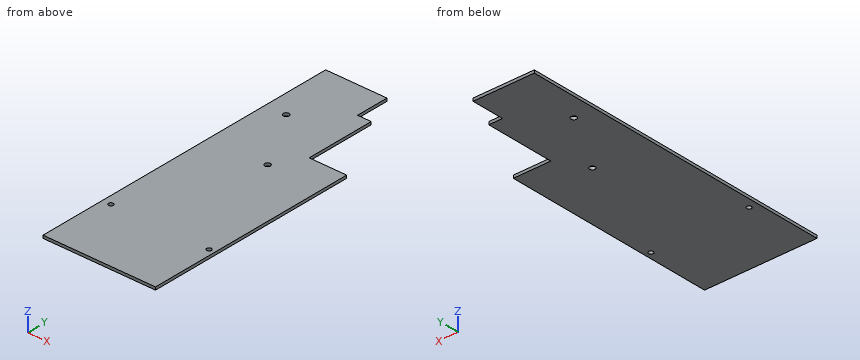
from build123d import *

# Parameters (mm, degrees)
RESSALTO_EXTRUS_O1_DEPTH                   = 1.5
CORTE_EXTRUS_O2_REACH                      = 167.453
ESBO_O5_R                                  = 1.5
BROCA_DE_ROSQUEAR_PARA_TARRAXA_DE_M3X0_5_D = 2.5
CORTE_EXTRUS_O3_REACH                      = 167.453
ESBO_O15_R                                 = 1.5
CORTE_EXTRUS_O4_REACH                      = 167.453
ESBO_O16_W                                 = 7.289764361
ESBO_O16_H                                 = 17.697498775


with BuildPart() as part:
    # Esboço2 → Ressalto-extrusão1 (new body)
    with BuildSketch(Plane(origin=(0, 0, 25.401562241), x_dir=(-1, 0, 0), z_dir=(0, 0, -1))):
        Polygon((40, 9.462441068), (0, 9.462441068), (0, -45.537558932), (-20, -45.537558932), (-20, -160.537558932), (40, -160.537558932), align=None)
    extrude(amount=RESSALTO_EXTRUS_O1_DEPTH)

    # Esboço5 → Corte-extrusão2 (cut, up to next)
    with BuildSketch(Plane(origin=(0, 0, 23.901562241), x_dir=(-1, 0, 0), z_dir=(0, 0, -1)), mode=Mode.PRIVATE) as corte_extrus_o2_sk1:
        with Locations((28.9, -26.787558932)):
            Circle(ESBO_O5_R)
    corte_extrus_o2_tool1 = extrude(corte_extrus_o2_sk1.sketch, amount=-CORTE_EXTRUS_O2_REACH, mode=Mode.PRIVATE) & part.part
    add(corte_extrus_o2_tool1.solids().sort_by_distance((-28.9, -26.787559, 23.901562))[0], mode=Mode.SUBTRACT)

    # Broca de rosquear para tarraxa de M3x0.52 (through all)
    with Locations(Plane(origin=(0, 0, 23.901562241), x_dir=(-1, 0, 0), z_dir=(0, 0, -1))):
        with Locations((-16.849169709, -124.734682683), (35.5, -124.808922584)):
            Hole(BROCA_DE_ROSQUEAR_PARA_TARRAXA_DE_M3X0_5_D / 2)

    # Esboço15 → Corte-extrusão3 (cut, up to next)
    with BuildSketch(Plane(origin=(0, 0, 23.901562241), x_dir=(-1, 0, 0), z_dir=(0, 0, -1)), mode=Mode.PRIVATE) as corte_extrus_o3_sk1:
        with Locations((8.9, -60.537558932)):
            Circle(ESBO_O15_R)
    corte_extrus_o3_tool1 = extrude(corte_extrus_o3_sk1.sketch, amount=-CORTE_EXTRUS_O3_REACH, mode=Mode.PRIVATE) & part.part
    add(corte_extrus_o3_tool1.solids().sort_by_distance((-8.9, -60.537559, 23.901562))[0], mode=Mode.SUBTRACT)

    # Esboço16 → Corte-extrusão4 (cut, up to next)
    with BuildSketch(Plane(origin=(0, 0, 23.901562241), x_dir=(-1, 0, 0), z_dir=(0, 0, -1)), mode=Mode.PRIVATE) as corte_extrus_o4_sk1:
        with Locations((3.644882181, 0.61369168)):
            Rectangle(ESBO_O16_W, ESBO_O16_H)
    corte_extrus_o4_tool1 = extrude(corte_extrus_o4_sk1.sketch, amount=-CORTE_EXTRUS_O4_REACH, mode=Mode.PRIVATE) & part.part
    add(corte_extrus_o4_tool1.solids().sort_by_distance((-3.644882, 0.613692, 23.901562))[0], mode=Mode.SUBTRACT)


solid = part.part
Work out the finished part from the listing and answer in its coordinate system (mm). Round coordinates to 2 decimals unless told otherwise and drop trailing zeros. Write each loop counter-clockwise with the first axis right and the second up, starting at its lowest first coordinate (ties: lowest second). Pieces come first, ordered by that corner, then holes. Notation, with made-up numbers: (-39, -34.5) -> (-10, -34.5) arc R13 cw to (-10, -27.5) -> close; hole circle Ø8 at (-34.75, 3). An arc over 180 degrees is marked (long way). Answer as CSV lines item,"result". Start each with the question number.
(1) The part is cut by section C-C, the plane y = -18.5. Give the vertices of the cut face in (x, z), then the cut area to 3 significant figures.
(2) Each of these flat-tipped pins is pushed along its axis until it touches: pin 1 (0.8 mm diameter, centred on x = 7, z = 24.5, fed in from +Y); pin 2 (2 mm diameter, centred on x = 16.85, y = -124.73, fed in from +Z). Where does it stop, or does it pass through?
(3) The part is cut by section A-A, the plane x = -28.9. Give the vertices of the cut face in (y, z).
(4) Find the intervals of material crossed by probe 1 along Y at (x, z) = (-28.9, 24.4); probe 2 along Y at (x, z) = (-35.5, 24.4); probe 3 along Y at (x, z) = (-7, 24.55), in increasing order.
(5) The part is cut by section B-B, the plane z = 24.3. Give the vertices of the cut face in (x, y), then the cut area to 3 significant figures.
Output values:
1,outline,"(-40, 23.9) -> (0, 23.9) -> (0, 25.4) -> (-40, 25.4) -> close"
1,area,"60.0 mm²"
2,pin 1,"stops at y = -45.54"
2,pin 2,"passes through"
3,outline,"(-160.54, 23.9) -> (-28.29, 23.9) -> (-28.29, 25.4) -> (-160.54, 25.4) -> close; (-25.29, 23.9) -> (9.46, 23.9) -> (9.46, 25.4) -> (-25.29, 25.4) -> close"
4,probe 1,"y = -160.54 to -28.29, -25.29 to 9.46"
4,probe 2,"y = -160.54 to -126.06, -123.56 to 9.46"
4,probe 3,"y = -160.54 to -8.24"
5,outline,"(-40, -160.54) -> (20, -160.54) -> (20, -45.54) -> (0, -45.54) -> (0, -8.24) -> (-7.29, -8.24) -> (-7.29, 9.46) -> (-40, 9.46) -> close; hole circle Ø2.5 at (-35.5, -124.81); hole circle Ø3 at (-28.9, -26.79); hole circle Ø3 at (-8.9, -60.54); hole circle Ø2.5 at (16.85, -124.73)"
5,area,"8,950 mm²"
